Model file for the job. Use its own axes, mm. Face numbers are marked on the shaded views. A direction names the side the tool comes from. Round coordinates to 2 decimals unless told otherwise and drop trailing zeros. Write each loop counter-clockwise with the first axis right and the second up, starting at its lowest first coordinate (ties: lowest second). Pieces come first, ordered by that corner, then holes. Notation, with made-up numbers: (2, 83) - (47, 83) arc R32 cw to (47, 121) - close; hole circle Ø7 at (29.25, 49). An arc over 180 degrees is marked (long way). Answer as a JSON object with one key per item and string values. Group by question number.
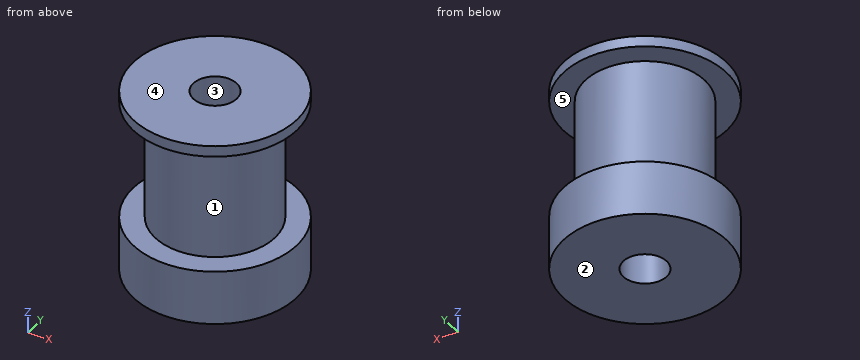
Autodesk Inventor part; units mm, degrees
ref_plane "YZ Plane" through (0, 0, 0) normal (1, 0, 0) x (0, 1, 0)
ref_plane "XZ Plane" through (0, 0, 0) normal (0, 1, 0) x (-1, 0, 0)
ref_plane "XY Plane" through (0, 0, 0) normal (0, 0, 1) x (1, 0, 0)
sketch "Skizze1" plane through (0, 0, 0) normal (0, 0, 1) x (1, 0, 0)
  circle A0 centre (0, 0) radius 7.5
  circle A1 centre (0, 0) radius 5.5
  circle A2 centre (0, 0) radius 2
  dimension "d0" = 15
  dimension "d3" = 11
  dimension "d9" = 4
extrude "Extrusion2" add sketch "Skizze1" against normal blind 11 contours A1 | A2
sketch "Skizze2" plane through (0, 0, -11) normal (0, 0, -1) x (-1, 0, 0)
  circle A0 centre (0, 0) radius 7.5
  dimension "d6" = 15
extrude "Extrusion3" add sketch "Skizze2" along normal blind 5
extrude "Extrusion4" cut sketch "Skizze1" along normal mid plane 50 contours A2
extrude "Extrusion5" add sketch "Skizze1" along normal blind 1 contours A0 | A1
properties part number "Timing belt pulley"
(1) Slice it at A-A (y = 0). Write the cut outline in (x, z), then the cut area to 3 significant figures.
(2) 3-axis set-ups, long thin cutter, end or side, ignore diameter. For the marked faces 4 and 5: which of +Z, -Z, +X, -X, +Y, -Y reach the whole face in a straight line?
(3) Slice it at C-C (z = -14.25). Write the cut outline in (x, y), then the cut area to 3 significant figures.
(4) Pull direction X, two halves, no side cores. Call the marked faces 1, 2 and 3: pulls with the +X half, pulls with the -X half, needs draft (parallel to the pull), parting line crosses it, or undercut.
(5) Flat gauge pins, fed straight in: pin 1 (1.5 mm diameter, centred on x = -6, z = -12, fed in from +Y); pin 2 (4 mm diameter, centred on x = 3, z = -5.5, fed in from -Y); pin 3 (2 mm diameter, centred on x = 0, z = -1.5, fed in from -Y). Where does each tip first touch, or does it go through?
(6) Drill centre lines: line 1 (Y direction, x = 0, z = -4.75); line 2 (Y direction, x = 0, z = -11.75); line 3 (Z direction, x = 5.25, y = 1.75). Where is each one in solid material? Low to high. Write a range as from..to.
(7) Slice it at D-D (x = -3.25). Write the cut outline in (y, z).
Answer:
{
 "1": {"outline": "(-7.5, -16) - (-2, -16) - (-2, 1) - (-7.5, 1) - (-7.5, 0) - (-5.5, 0) - (-5.5, -11) - (-7.5, -11) - close; (2, -16) - (7.5, -16) - (7.5, -11) - (5.5, -11) - (5.5, 0) - (7.5, 0) - (7.5, 1) - (2, 1) - close", "area": "143 mm²"},
 "2": {"face 4": "+Z, +X, -X, +Y, -Y", "face 5": "none"},
 "3": {"outline": "circle Ø15 at (0, 0); hole circle Ø4 at (0, 0)", "area": "164 mm²"},
 "4": {"face 1": "parting line crosses it", "face 2": "needs draft", "face 3": "undercut"},
 "5": {"pin 1": "y = 5.36", "pin 2": "y = -5.41", "pin 3": "y = -5.5"},
 "6": {"line 1": "-5.5..-2, 2..5.5", "line 2": "-7.5..-2, 2..7.5", "line 3": "-16..-11, 0..1"},
 "7": {"outline": "(-6.76, -16) - (6.76, -16) - (6.76, -11) - (4.44, -11) - (4.44, 0) - (6.76, 0) - (6.76, 1) - (-6.76, 1) - (-6.76, 0) - (-4.44, 0) - (-4.44, -11) - (-6.76, -11) - close"}
}
